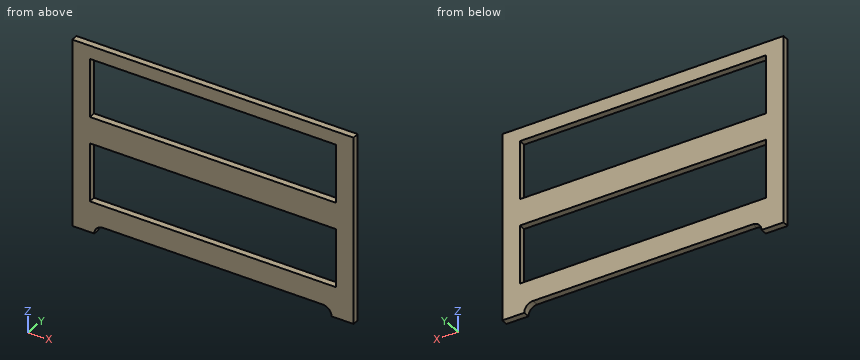
```python
from build123d import *

# Parameters (mm, degrees)
F0_W     = 812.8
F0_H     = 488.95
F0_W_2   = 711.2
F0_H_2   = 168.275
F1_DEPTH = 19.05


with BuildPart() as f1:
    # F0 (on Front) → F1 (new body)
    with BuildSketch(Plane.XZ):
        with BuildLine():
            Line((812.8, 0), (0, 0))
            Line((0, 0), (0, -50.8))
            Line((0, -50.8), (63.5, -50.8))
            ThreePointArc((63.5, -50.8), (70.939488, -32.839488), (88.9, -25.4))
            Line((88.9, -25.4), (406.4, -25.4))
            Line((406.4, -25.4), (723.9, -25.4))
            ThreePointArc((723.9, -25.4), (741.860512, -32.839488), (749.3, -50.8))
            Line((749.3, -50.8), (812.8, -50.8))
            Line((812.8, -50.8), (812.8, 0))
        make_face()
        with Locations((406.4, 244.475)):
            Rectangle(F0_W, F0_H)
        with Locations((406.4, 122.2375)):
            Rectangle(F0_W_2, F0_H_2, mode=Mode.SUBTRACT)
        with Locations((406.4, 366.7125)):
            Rectangle(F0_W_2, F0_H_2, mode=Mode.SUBTRACT)
    extrude(amount=F1_DEPTH)


solid = f1.part
```
Model file for the job. Use its own axes, mm. Round coordinates to 2 decimals unless told otherwise and drop trailing zeros. Write each loop counter-clockwise with the first axis right and the second up, starting at its lowest first coordinate (ties: lowest second). Pieces come first, ordered by that corner, then holes. Notation, with made-up numbers: (-33, -10) -> (15, -10) arc R10 ccw to (15, 8) -> close; hole circle Ø4 at (43.25, -27). An arc over 180 degrees is marked (long way). Answer as CSV lines item,"result".
1. Pin check, flat tip, straight feed: pin 1 Ø9.5 at (x, y) = (356.5, -12) entering from -Z. Stop position of the tip, or through.
Resolved:
pin 1,"z = -25.4"
2. Slice it at A-A, the plane z = 432. List the corners of the cut face in (x, y), plus the area to 3 significant figures.
Resolved:
outline,"(0, -19.05) -> (50.8, -19.05) -> (50.8, 0) -> (0, 0) -> close; (762, -19.05) -> (812.8, -19.05) -> (812.8, 0) -> (762, 0) -> close"
area,"1,940 mm²"
3. Slice it at B-B, the plane x = 646.5. List the corners of the cut face in (y, z) (3 decimals), plus the area to 3 significant figures.
Resolved:
outline,"(-19.05, -25.4) -> (0, -25.4) -> (0, 38.1) -> (-19.05, 38.1) -> close; (-19.05, 206.375) -> (0, 206.375) -> (0, 282.575) -> (-19.05, 282.575) -> close; (-19.05, 450.85) -> (0, 450.85) -> (0, 488.95) -> (-19.05, 488.95) -> close"
area,"3,390 mm²"
4. Slice it at C-C, the plane y = -14.5. List the corners of the cut face in (x, z) (3 decimals).
Resolved:
outline,"(0, -50.8) -> (63.5, -50.8) arc R25.4 cw to (88.9, -25.4) -> (723.9, -25.4) arc R25.4 cw to (749.3, -50.8) -> (812.8, -50.8) -> (812.8, 488.95) -> (0, 488.95) -> close; hole (50.8, 38.1) -> (762, 38.1) -> (762, 206.375) -> (50.8, 206.375) -> close; hole (50.8, 282.575) -> (762, 282.575) -> (762, 450.85) -> (50.8, 450.85) -> close"
5. Drill centre lines: line 1 (Z direction, x = 649.5, y = -8.5) (3 decimals); line 2 (Z direction, x = 743, y = -12.75) (3 decimals); line 3 (X direction, y = -0.75, z = 405). Where is each one in solid material? Low to high.
Resolved:
line 1,"-25.4 to 38.1, 206.375 to 282.575, 450.85 to 488.95"
line 2,"-34.056 to 38.1, 206.375 to 282.575, 450.85 to 488.95"
line 3,"0 to 50.8, 762 to 812.8"
